Autodesk Inventor part; units mm, degrees
ref_plane "YZ Plane" through (0, 0, 0) normal (1, 0, 0) x (0, 1, 0)
ref_plane "XZ Plane" through (0, 0, 0) normal (0, 1, 0) x (-1, 0, 0)
ref_plane "XY Plane" through (0, 0, 0) normal (0, 0, 1) x (1, 0, 0)
sketch "Sketch1" plane through (0, 0, 0) normal (0, 1, 0) x (-1, 0, 0)
  line L0 (0, 0) -> (-24, 0)
  line L1 (-24, 0) -> (-24, -46)
  line L2 (-24, -46) -> (0, -46)
  line L3 (0, -46) -> (0, 0)
  dimension "d0" = 24
  dimension "d1" = 46
extrude "Extrusion1" add sketch "Sketch1" along normal blind 23
sketch "Sketch2" plane through (0, 23, 0) normal (0, 1, 0) x (1, 0, 0)
  line L0 (4.75, 0) -> (19.25, 0)
  line L1 (19.25, 0) -> (19.25, 5)
  line L2 (19.25, 23) -> (4.75, 23)
  line L3 (4.75, 5) -> (4.75, 0)
  line L4 (4.75, 0) -> (19.25, 23) construction
  line L5 (19.25, 0) -> (4.75, 23) construction
  line L6 (0, 0) -> (24, 0)
  arc A0 (13, 23) -> (11, 23) centre (12, 23) ccw
  arc A1 (4.75, 23) -> (4.75, 5) centre (10.9013, 14) ccw
  line L7 (0, 46) -> (0, 0)
  arc A2 (19.25, 5) -> (19.25, 23) centre (13.0987, 14) ccw
  line L8 (24, 0) -> (24, 46)
  circle A3 centre (12, 34) radius 4.5
  line L9 (24, 46) -> (0, 46)
  point P0 (12, 11.5)
  point P1 (12, 0)
  dimension "d4" = 14.5
  dimension "d5" = 23
  dimension "d6" = 2
  dimension "d8" = 9
  dimension "d9" = 12
extrude "Extrusion2" add sketch "Sketch2" along normal blind 2 contours A0 L2 | A3
extrude "Extrusion3" add sketch "Sketch2" along normal blind 8 contours L3 A1 L2 A2 L1 L0
sketch "Sketch3" plane through (0, 31, 0) normal (0, 1, 0) x (1, 0, 0)
  line L0 (17.25, 6.5) -> (6.75, 6.5)
  line L1 (6.75, 21.5) -> (17.25, 21.5)
  line L2 (17.25, 6.5) -> (6.75, 21.5) construction
  line L3 (6.75, 6.5) -> (17.25, 21.5) construction
  line L4 (19.25, 23) -> (4.75, 23)
  arc A0 (6.75, 21.5) -> (6.75, 6.5) centre (10.8385, 14) ccw
  arc A1 (17.25, 6.5) -> (17.25, 21.5) centre (13.1615, 14) ccw
  point P0 (0, 0)
  point P1 (12, 14)
  dimension "d17" = 8.542
  dimension "d18" = 8.542
extrude "Extrusion4" add sketch "Sketch3" along normal blind 24
sketch "Sketch4" plane through (0, 55, 0) normal (0, 1, 0) x (1, 0, 0)
  circle A0 centre (12, 14) radius 3
  line L0 (17.25, 21.5) -> (6.75, 21.5)
  line L1 (6.75, 6.5) -> (17.25, 6.5)
  point P0 (0, 0)
  dimension "d21" = 6
  dimension "d22" = 7.5
  dimension "d23" = 15
extrude "Extrusion5" add sketch "Sketch4" along normal blind 2
sketch "Sketch5" plane through (24, 0, 0) normal (1, 0, 0) x (0, 0, -1)
  circle A0 centre (42, 4) radius 2
  line L0 (46, 0) -> (46, 23)
  line L1 (0, 0) -> (46, 0)
  circle A1 centre (26, 4) radius 2
  dimension "d26" = 4
  dimension "d27" = 4
  dimension "d28" = 4
  dimension "d29" = 4
  dimension "d30" = 16
extrude "Extrusion6" cut sketch "Sketch5" against normal blind 10
sketch "Sketch6" plane through (0, 0, -46) normal (-1, 0, 0) x (0, 0, 1)
  circle A0 centre (4, 4) radius 2
  circle A1 centre (4, 4) radius 2
  circle A2 centre (20, 4) radius 2
  circle A3 centre (20, 4) radius 2
  point P0 (46, 0)
extrude "Extrusion7" cut sketch "Sketch6" against normal blind 10
sketch "Sketch7" plane through (0, 0, 0) normal (0, -1, 0) x (1, 0, 0)
  circle A0 centre (20, -10) radius 2
  line L0 (24, 0) -> (24, -46)
  line L1 (0, 0) -> (24, 0)
  circle A1 centre (4, -10) radius 2
  line L2 (0, -46) -> (0, 0)
  circle A2 centre (12, -34) radius 2.5
  line L3 (24, -46) -> (0, -46)
  point P0 (12, -46)
  dimension "d35" = 4
  dimension "d36" = 4
  dimension "d37" = 10
  dimension "d38" = 4
  dimension "d39" = 4
  dimension "d40" = 5
  dimension "d41" = 12
extrude "Extrusion8" cut sketch "Sketch7" against normal blind 10 contours A0 | A1
extrude "Extrusion9" add sketch "Sketch7" along normal blind 2 contours A2
sketch "Sketch8" plane through (12, -2, -34) normal (0, -1, 0) x (1, 0, 0)
  circle A0 centre (0, 0) radius 2.5
  line L0 (1.75, -1.7854) -> (-1.75, -1.7854)
  line L1 (-1.75, -1.7854) -> (-1.75, 1.7854)
  line L2 (-1.75, 1.7854) -> (1.75, 1.7854)
  line L3 (1.75, 1.7854) -> (1.75, -1.7854)
  line L4 (1.75, -1.7854) -> (-1.75, 1.7854) construction
  line L5 (-1.75, -1.7854) -> (1.75, 1.7854) construction
  arc A1 (-1.75, -1.7854) -> (1.75, -1.7854) centre (0, 0) ccw
  arc A2 (1.75, 1.7854) -> (-1.75, 1.7854) centre (0, 0) ccw
  point P0 (-12, 34)
  point P1 (-1.75, -1.7854)
  point P2 (1.75, 1.7854)
  dimension "d46" = 3.5
  dimension "d47" = 3.5707
extrude "Extrusion10" add sketch "Sketch8" along normal blind 7 contours L2 A0 | L3 L0 L1 L2 | A0 L0
properties part number "Encoder Motor"
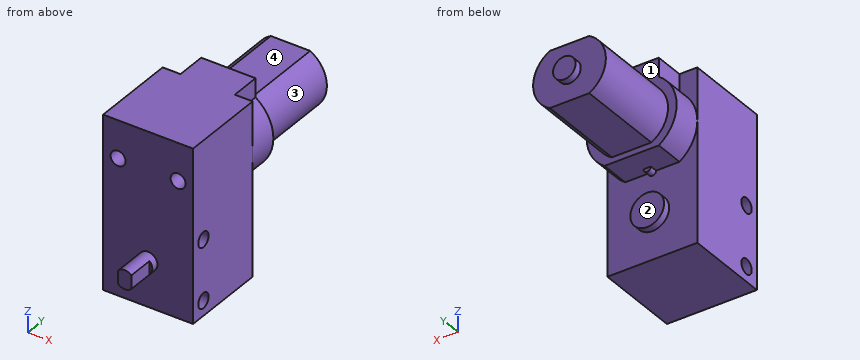
Design review of the part built by this model. Coordinates are the model's own, in mm. Face numbers are marked on the shaded views. A direction names the side the tool comes from. Round coordinates to 2 decimals unless told otherwise and drop trailing zeros. Order: outer loops, then holes, each group sorted by start corner. A loop starts at its lowest first (then second) coordinate and runs counter-clockwise, first axis right, second up. Notation, with made-up numbers: M 59,76 L 82,76 A19 ccw 82,84 Z; hole C 36,-10.75 d9. An arc over 180 degrees is marked long. Answer as CSV lines item,"result". Start each with the question number.
1) Add section D-D (x = 20). Give the boundary of the cut face in (y, z).
2) For pin 1 Ø3 at (y, z) = (4, -42) entering from +X; pin 2 Ø5 at (x, z) = (2.5, -8) entering from +Y; pin 3 Ø1.1 at (y, z) = (-7, -34.5) entering from +X; pin 4 Ø1.5 at (y, z) = (44.5, -23) entering from -X, all flat-tipped, find the tip position at first contact; note any pin that passes through.
3) Add section C-C (z = -26). Give the boundary of the cut face in (x, y).
4) Add section A-A (y = 4). Give the boundary of the cut face in (x, z), then the cut area to 3 significant figures.
5) Wall thickness on line 1 along Y through (x, z) = (17.25, -26); line 2 along Y through (x, z) = (1.5, -35); line 3 along Z through (x, y) = (4, 6.5): over which ranges is each line inside the solid? List them lowest first. Write a range as [from, to].
6) Tool access review of the marked faces 1, 2, 3 and 4: name each direction out of +Z, -Z, +X, -X, +Y, -Y from which nothing blocks a thin tool from reaching the whole face with its end or side.
7) Add section B-B (x = 12). Give the boundary of the cut face in (y, z), then the cut area to 3 significant figures.
Resolved:
1,outline,"M 0,-46 L 23,-46 L 23,-22.44 L 31,-22.44 L 31,-19.12 L 55,-19.12 L 55,-8.88 L 31,-8.88 L 31,-5.56 L 23,-5.56 L 23,0 L 0,0 L 0,-8 L 10,-8 L 10,-12 L 0,-12 Z; hole C 4,-42 d4; hole C 4,-26 d4"
2,pin 1,"x = 14"
2,pin 2,"y = 55"
2,pin 3,"x = 13.75"
2,pin 4,"through"
3,outline,"M 0,0 L 24,0 L 24,2 L 14,2 L 14,6 L 24,6 L 24,23 L 0,23 L 0,6 L 10,6 L 10,2 L 0,2 Z"
4,outline,"M 0,-46 L 24,-46 L 24,-44 L 14,-44 L 14,-40 L 24,-40 L 24,-28 L 14,-28 L 14,-24 L 24,-24 L 24,0 L 0,0 L 0,-24 L 10,-24 L 10,-28 L 0,-28 L 0,-40 L 10,-40 L 10,-44 L 0,-44 Z; hole C 4,-10 d4; hole C 20,-10 d4"
4,area,"919 mm^2"
5,line 1,"[0, 2], [6, 23]"
5,line 2,"[0, 23]"
5,line 3,"[-46, -12], [-8, 0]"
6,face 1,"+Y"
6,face 2,"-Z, +X, -X, +Y"
6,face 3,"+X, +Y"
6,face 4,"+Z, +X, -X, +Y"
7,outline,"M -9,-36.5 L 0,-36.5 L 0,-46 L 23,-46 L 23,-38.5 L 25,-38.5 L 25,-29.5 L 23,-29.5 L 23,-24 L 25,-24 L 25,-23 L 31,-23 L 31,-21.5 L 55,-21.5 L 55,-17 L 57,-17 L 57,-11 L 55,-11 L 55,-6.5 L 31,-6.5 L 31,0 L 0,0 L 0,-31.5 L -9,-31.5 Z"
7,area,"1,680 mm^2"
